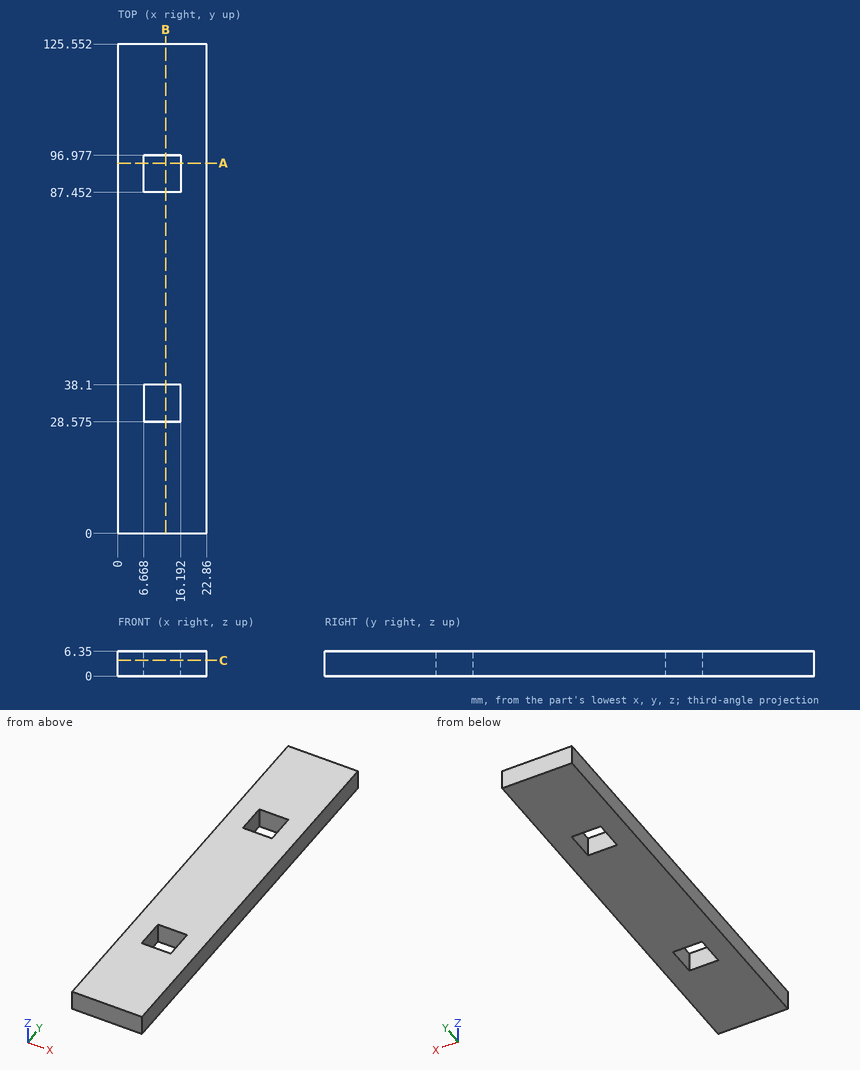
Study the drawing (mm; zero at the part's minimum x, y, z) and answer. Round coordinates to 2 decimals unless told otherwise and drop trailing zeros. Write each loop counter-clockwise with the first axis right and the second up, starting at its lowest first coordinate (ties: lowest second). Pieces come first, ordered by that corner, then holes. Notation, with made-up numbers: (44, 43) - (62, 43) arc R10 cw to (62, 48) - close; hole circle Ø1 at (39, -20). An arc over 180 degrees is marked (long way). Use a Markdown table: item, result. Add a question column.
1. Consider line 1 (Y direction, x = 9, z = 3.5) (1 decimal); line 2 (X direction, y = 33, z = 3.25). Determine where each line is inside the solid, lowest interval first.
2. The part is cut by section B-B (x = 12.25). Give the number of separate pieces and of enclosed holes in the cut face.
3. The part is cut by section C-C (z = 4). Write down the section's boundary in (x, y) (1 decimal).
4. The part is cut by section A-A (y = 95). Write down the section's boundary in (x, z).
Reported:
| question | item | result |
|---|---|---|
| 1 | line 1 | 0 to 28.6, 38.1 to 87.5, 97 to 125.6 |
| 1 | line 2 | 0 to 6.67, 16.19 to 22.86 |
| 2 | separate pieces | 3 |
| 2 | enclosed holes | 0 |
| 3 | outline | (0, 0) - (22.9, 0) - (22.9, 125.6) - (0, 125.6) - close; hole (6.7, 28.6) - (16.2, 28.6) - (16.2, 38.1) - (6.7, 38.1) - close; hole (6.7, 87.5) - (16.2, 87.5) - (16.2, 97) - (6.7, 97) - close |
| 4 | outline | (0, 0) - (6.67, 0) - (6.67, 6.35) - (0, 6.35) - close; (16.19, 0) - (22.86, 0) - (22.86, 6.35) - (16.19, 6.35) - close |
